Check sheet for the modelled part. Datum: model origin and axes. Units: mm. A direction names the side the tool comes from. Round coordinates to 2 decimals unless told otherwise and drop trailing zeros. Write each loop counter-clockwise with the first axis right and the second up, starting at its lowest first coordinate (ties: lowest second). Pieces come first, ordered by that corner, then holes.
Item 1: Tool access check on faces 4 (the cylindrical face through (5.52, 20.24, -3.14)), 5 (the flat face through (8, 91.85, 0)), 6 (the cylindrical face through (-6.491, 117.902, -8.466)), 7 (the flat face through (-5, 125, 5)), 8 (the cylindrical face through (6.491, 10.846, -8.466)). Record the directions out of +Z, -Z, +X, -X, +Y, -Y that give a thin tool (end or side, any length) a straight path to the whole face; none if there is none.
Item 2: Cross-section at D-D on x = -9. Enter the section's corners in (y, z), plus the area to 3 significant figures.
Item 3: Material ranges on line 1 (Y direction, x = 7.5, z = 1.5); line 2 (Y direction, x = 9.75, z = 4.75); line 3 (Z direction, x = -0.5, y = 42), recorded low to high.
Item 4: Go/stop test with flat-tipped pins: pin 1 Ø8 at (x, z) = (1.5, -4.5) entering from -Y; pin 2 Ø1.1 at (y, z) = (61, 0) entering from +X; pin 3 Ø1 at (x, y) = (2.5, 19) entering from -Z; pin 4 Ø0.6 at (x, y) = (6.5, 104) entering from -Z. Record where each tip stops, or that it passes through.
Item 5: Cross-section at B-B on z = 3. Enter the section's corners in (x, y), plus the area to 3 significant figures.
Item 6: Release check for a two-part mould opening along Z. For faces 1 (the flat face through (8, 41.05, 0)), 2 (the cylindrical face through (-10.85, 65.88, -2.41)), 3 (the cylindrical face through (5.52, 108.19, -3.14)) record: +Z half, -Z half, draft (parallel to the pull), parting line (faces both ways), or undercut.
from build123d import *

# Parameters (mm, degrees)
SKETCH1_R               = 11.1125
SKETCH1_R_2             = 6.35
BOSS_EXTRUDE1_DEPTH     = 125
CUT_EXTRUDE1_START      = -14
SKETCH2_R               = 11.1125
SKETCH2_R_2             = 10.668
CUT_EXTRUDE1_DEPTH      = 14
SKETCH3_R               = 11.1125
SKETCH3_R_2             = 10.668
CUT_EXTRUDE2_DEPTH      = 22
CUT_EXTRUDE3_DEPTH      = 126.984028006
CUT_EXTRUDE3_DEPTH_BACK = 126.984028006
SKETCH4_W               = 11.1125
SKETCH4_H               = 50.8
SKETCH6_W               = 0.5
SKETCH6_H               = 1
CUT_EXTRUDE4_DEPTH      = 126.984028006
CIRPATTERN1_COUNT       = 6


with BuildPart() as part:
    # Sketch1 → Boss-Extrude1 (new body)
    with BuildSketch(Plane(origin=(0, 0, 0), x_dir=(1, 0, 0), z_dir=(0, 1, 0))):
        with Locations(Location((0, 0, 0), (0, 0, 270))):
            Circle(SKETCH1_R)
        with Locations(Location((0, 0, 0), (0, 0, 270))):
            Circle(SKETCH1_R_2, mode=Mode.SUBTRACT)
    extrude(amount=BOSS_EXTRUDE1_DEPTH)

    # Sketch2 → Cut-Extrude1 (cut)
    with BuildSketch(Plane(origin=(0, 125, 0), x_dir=(1, 0, 0), z_dir=(0, 1, 0)).offset(CUT_EXTRUDE1_START)):
        with Locations(Location((0, 0, 0), (0, 0, 270))):
            Circle(SKETCH2_R)
        with Locations(Location((0, 0, 0), (0, 0, 270))):
            Circle(SKETCH2_R_2, mode=Mode.SUBTRACT)
    extrude(amount=CUT_EXTRUDE1_DEPTH, mode=Mode.SUBTRACT)

    # Sketch3 → Cut-Extrude2 (cut)
    with BuildSketch(Plane.XZ):
        with Locations(Location((0, 0, 0), (0, 0, 270))):
            Circle(SKETCH3_R)
        with Locations(Location((0, 0, 0), (0, 0, 90))):
            Circle(SKETCH3_R_2, mode=Mode.SUBTRACT)
    extrude(amount=-CUT_EXTRUDE2_DEPTH, mode=Mode.SUBTRACT)

    # Sketch4 → Cut-Extrude3 (cut, two sides: drawn at the far end of the back side and taken through both)
    with BuildSketch(Plane.XY.offset(-CUT_EXTRUDE3_DEPTH_BACK)):
        with Locations((5.55625, 66.45)):
            Rectangle(SKETCH4_W, SKETCH4_H)
    extrude(amount=CUT_EXTRUDE3_DEPTH + CUT_EXTRUDE3_DEPTH_BACK, mode=Mode.SUBTRACT)

    # Sketch6 → Cut-Extrude4 (cut, through all)
    with BuildSketch(Plane.XZ):
        with Locations((-6.580284354, 0)):
            Rectangle(SKETCH6_W, SKETCH6_H)
    cut_extrude4 = extrude(amount=-CUT_EXTRUDE4_DEPTH, mode=Mode.SUBTRACT)

    # CirPattern1: Cut-Extrude4 ×6 about axis
    cirpattern1_axis = Axis((0, 0, 0), (0, 1, 0))
    for i in range(1, CIRPATTERN1_COUNT):
        add(cut_extrude4.rotate(cirpattern1_axis, i * 360 / CIRPATTERN1_COUNT), mode=Mode.SUBTRACT)


solid = part.part
Response values:
1. face 4: +Y, -Y
1. face 5: +Z, -Z, +X
1. face 6: +Y
1. face 7: +Z, -Z, +X, -X, +Y
1. face 8: -Y
2. outline: (0, -5.73) - (22, -5.73) - (22, -6.52) - (111, -6.52) - (111, -5.73) - (125, -5.73) - (125, 5.73) - (111, 5.73) - (111, 6.52) - (22, 6.52) - (22, 5.73) - (0, 5.73) - close
2. area: 1,570 mm2
3. line 1: y = 0 to 41.05, 91.85 to 125
3. line 2: y = 22 to 41.05, 91.85 to 111
3. line 3: z = -11.1 to -6.33, 6.33 to 11.1
4. pin 1: stops at y = 0
4. pin 2: stops at x = -6.33
4. pin 3: stops at z = -10.48
4. pin 4: stops at z = -9.22
5. outline: (-10.7, 22) - (-10.24, 22) - (-10.24, 0) - (-5.6, 0) - (-5.6, 125) - (-10.24, 125) - (-10.24, 111) - (-10.7, 111) - close; (5.6, 0) - (10.24, 0) - (10.24, 22) - (10.7, 22) - (10.7, 41.05) - (5.6, 41.05) - close; (5.6, 91.85) - (10.7, 91.85) - (10.7, 111) - (10.24, 111) - (10.24, 125) - (5.6, 125) - close
5. area: 983 mm2
6. face 1: draft
6. face 2: parting line
6. face 3: undercut
